Geometry: see drawing. Coordinates: mm, zero at the bounding-box minimum. Coordinates: 2 decimals unless noted, no trailing zeros. Order: outer loops, then holes, each group sorted by start corner. A loop starts at its lowest first (then second) coordinate and runs counter-clockwise, first axis right, second up.
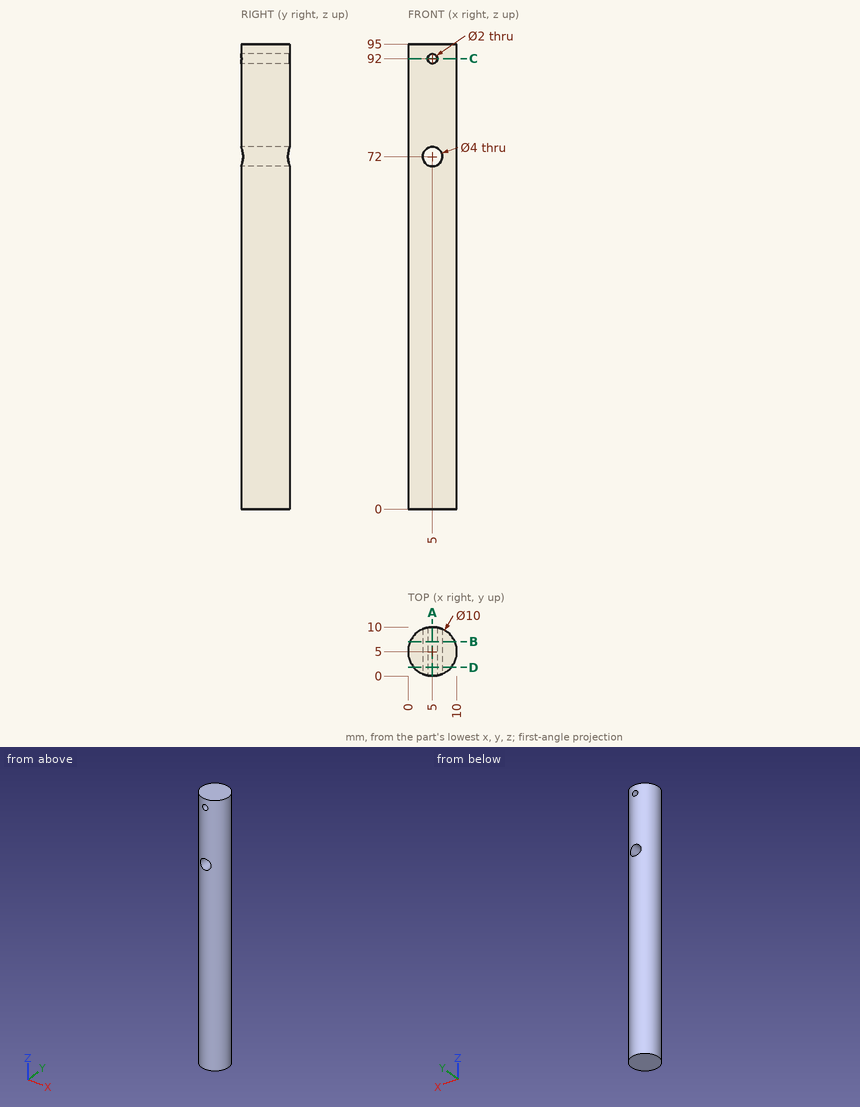
Q1. Section query A-A on x = 5. Output: boundary loops of the cut face in (y, z).
Solutions:
outline: (0, 0) - (10, 0) - (10, 70) - (0, 70) - close; (0, 74) - (10, 74) - (10, 91) - (0, 91) - close; (0, 93) - (10, 93) - (10, 95) - (0, 95) - close
Q2. Section query B-B on y = 7. Output: boundary loops of the cut face in (x, z).
Solutions:
outline: (0.42, 0) - (9.58, 0) - (9.58, 95) - (0.42, 95) - close; hole circle Ø4 at (5, 72); hole circle Ø2 at (5, 92)
Q3. Material intervals for line 1 along X through (y, z) = (4.75, 92); line 2 along Y through (x, z) = (5.25, 31); line 3 along Z through (x, y) = (5.5, 2.5), sorted ascending.
Solutions:
line 1: x = 0.01 to 4, 6 to 9.99
line 2: y = 0.01 to 9.99
line 3: z = 0 to 70.06, 73.94 to 91.13, 92.87 to 95
Q4. Section query D-D on y = 1.75. Output: boundary loops of the cut face in (x, z), plus the area to 3 significant figures.
Solutions:
outline: (1.2, 0) - (8.8, 0) - (8.8, 95) - (1.2, 95) - close; hole circle Ø4 at (5, 72); hole circle Ø2 at (5, 92)
area: 706 mm2
Q5. Section query C-C on z = 92. Output: boundary loops of the cut face in (x, y), plus the area to 3 significant figures.
Solutions:
outline: (4, 0.1) - (4, 9.9) arc R5 ccw to start; (6, 0.1) arc R5 ccw to (6, 9.9) - close
area: 58.7 mm2
Q6. Pin query (flat end, axial travel): P1, Ø2, axis at y = 1.5, z = 11, coming from the -X side; P2, Ø3, axis at y = 4.5, z = 39, coming from the +X side; P3, Ø1, axis at x = 2, z = 61, coming from the +Y side; P4, Ø1.8, axis at x = 5, z = 92, coming from the -Y side. Return the tip coordinate at first contact, or that it passes through.
Solutions:
P1: stops at x = 0.67
P2: stops at x = 10
P3: stops at y = 9.33
P4: passes through
